For this review, take the finished solid that the model builds, in its own axes (mm). A direction names the side the tool comes from. Round coordinates to 2 decimals unless told otherwise and drop trailing zeros. Loops run counter-clockwise (first coordinate to the right, second up) from the corner with the lowest first, then second, coordinate; pieces in that order, holes last.
```python
from build123d import *

# Parameters (mm, degrees)
SKETCH2_R           = 2.15
SKETCH2_R_2         = 5.565
BOSS_EXTRUDE1_DEPTH = 1.2
SKETCH3_W           = 12.7
SKETCH3_H           = 15.24
BOSS_EXTRUDE2_DEPTH = 35


with BuildPart() as part:
    # Sketch1 → Revolve1 (revolve)
    with BuildSketch(Plane(origin=(0, 0, 0), x_dir=(0, 0, -1), z_dir=(1, 0, 0))):
        Polygon((0, 0), (0, 2), (-1, 2), (-1, 27.5), (-24, 27.5), (-24, 5.565), (-27.2, 5.565), (-27.2, 2), (-38.2, 2), (-38.2, 0), align=None)
    revolve(axis=Axis((0, 0, 38.2), (0, 0, -1)))

    # Sketch2 → Boss-Extrude1 (add)
    with BuildSketch(Plane.XY.offset(24)):
        with BuildLine():
            Line((-17.440029985, 21.262534048), (-37.377061469, 4.909712407))
            ThreePointArc((-37.377061469, 4.909712407), (-39.692308695, 0.312442672), (-37.840128061, -4.490128061))
            Line((-37.840128061, -4.490128061), (-35.330256121, -7))
            Line((-35.330256121, -7), (-26.594172294, -7))
            ThreePointArc((-26.594172294, -7), (0, -27.5), (26.594172294, -7))
            Line((26.594172294, -7), (35.330256121, -7))
            Line((35.330256121, -7), (37.840128061, -4.490128061))
            ThreePointArc((37.840128061, -4.490128061), (39.692308695, 0.312442672), (37.377061469, 4.909712407))
            Line((37.377061469, 4.909712407), (17.440029985, 21.262534048))
            ThreePointArc((17.440029985, 21.262534048), (0, 27.5), (-17.440029985, 21.262534048))
        make_face()
        with Locations((-33.35, 0)):
            Circle(SKETCH2_R, mode=Mode.SUBTRACT)
        with Locations((33.35, 0)):
            Circle(SKETCH2_R, mode=Mode.SUBTRACT)
        Circle(SKETCH2_R_2, mode=Mode.SUBTRACT)
    extrude(amount=BOSS_EXTRUDE1_DEPTH)

    # Sketch3 → Boss-Extrude2 (add)
    with BuildSketch(Plane(origin=(0, 0, 0), x_dir=(1, 0, 0), z_dir=(0, 1, 0))):
        with Locations((0, -8.62)):
            Rectangle(SKETCH3_W, SKETCH3_H)
    extrude(amount=-BOSS_EXTRUDE2_DEPTH)


solid = part.part
```
(1) Insertion check: pin 1 Ø2.5 at (y, z) = (-31.5, 8) entering from +X; pin 2 Ø10 at (x, z) = (-19, 15.5) entering from -Y; pin 3 Ø2 at (x, z) = (22, 21.5) entering from +Y; pin 4 Ø4 at (x, y) = (-33.35, 0) entering from -Z. Each pin has a flat end and moves straight along its axis. Give the tip position at first contact, or say it passes through.
(2) For L1, parallel to Z at x = 24, y = 8.5; L2, parallel to Y at x = -7, z = 4; L3, parallel to Y at x = 33.35, z = 24.45, list the stretches that pass through material, from the lowest coordinate up.
(3) Add section A-A (y = 0). Give the boundary of the cut face in (x, z) (3 decimals).
(4) Add section C-C (x = -33.35). Give the boundary of the cut face in (y, z).
(5) Add section B-B (x = 0). Give the boundary of the cut face in (y, z) (3 decimals).
(6) Add section D-D (z = 21.5). Give the boundary of the cut face in (x, y).
(7) The part is to be moulded in two halves that separate along X. For faces 5 (the flat face through (0, -35, 9)), 6 (the cylindrical face through (-2.13, 5.14, 26.21)), 7 (the cylindrical face through (-31.3, 0.65, 24.59)), say which applies: pulls with the +X half, pulls with the -X half, needs draft (parallel to the pull), parting line crosses it, or undercut.
(8) For faces 1 (the flat face through (6.35, -31, 9)), 2 (the flat face through (-6.35, -31, 9)), 3 (the flat face through (0, 0, 0)), 4 (the cylindrical face through (-2, 0, 33)), list the 3-axis set-ups (+Z, -Z, +X, -X, +Y, -Y) from which the entire face can be reached by the end or side of a thin tool; tool diameter is ignored.
Outcome:
1. pin 1: stops at x = 6.35
1. pin 2: stops at y = -23.67
1. pin 3: stops at y = 17.76
1. pin 4: passes through
2. L1: z = 1 to 25.2
2. L2: y = -26.59 to 26.59
2. L3: y = -7 to -2.15, 2.15 to 8.21
3. outline: (-39.7, 24) - (-35.5, 24) - (-35.5, 25.2) - (-39.7, 25.2) - close; (-31.2, 24) - (-27.5, 24) - (-27.5, 1) - (-2, 1) - (-2, 0) - (2, 0) - (2, 1) - (27.5, 1) - (27.5, 24) - (31.2, 24) - (31.2, 25.2) - (5.565, 25.2) - (5.565, 27.2) - (2, 27.2) - (2, 38.2) - (-2, 38.2) - (-2, 27.2) - (-5.565, 27.2) - (-5.565, 25.2) - (-31.2, 25.2) - close; (35.5, 24) - (39.7, 24) - (39.7, 25.2) - (35.5, 25.2) - close
4. outline: (-7, 24) - (-2.15, 24) - (-2.15, 25.2) - (-7, 25.2) - close; (2.15, 24) - (8.21, 24) - (8.21, 25.2) - (2.15, 25.2) - close
5. outline: (-35, 1) - (-2, 1) - (-2, 0) - (2, 0) - (2, 1) - (27.5, 1) - (27.5, 25.2) - (5.565, 25.2) - (5.565, 27.2) - (2, 27.2) - (2, 38.2) - (-2, 38.2) - (-2, 27.2) - (-5.565, 27.2) - (-5.565, 25.2) - (-27.5, 25.2) - (-27.5, 16.24) - (-35, 16.24) - close
6. outline: circle Ø55 at (0, 0)
7. face 5: needs draft
7. face 6: parting line crosses it
7. face 7: undercut
8. face 1: +Z, -Z, +X, -Y
8. face 2: +Z, -Z, -X, -Y
8. face 3: -Z, +X, -X, +Y, -Y
8. face 4: +Z
